Verification items for this drawing (mm, ordinates from the low corner). A direction names the side the tool comes from. Round coordinates to 2 decimals unless told otherwise and drop trailing zeros. Loops run counter-clockwise (first coordinate to the right, second up) from the corner with the lowest first, then second, coordinate; pieces in that order, holes last. Notation, with made-up numbers: (31, 5.5) - (40, 5.5) arc R33 ccw to (40, 41.5) - close; hole circle Ø6 at (39, -13). An arc over 180 degrees is marked (long way). Put each result on its own line as item: value.
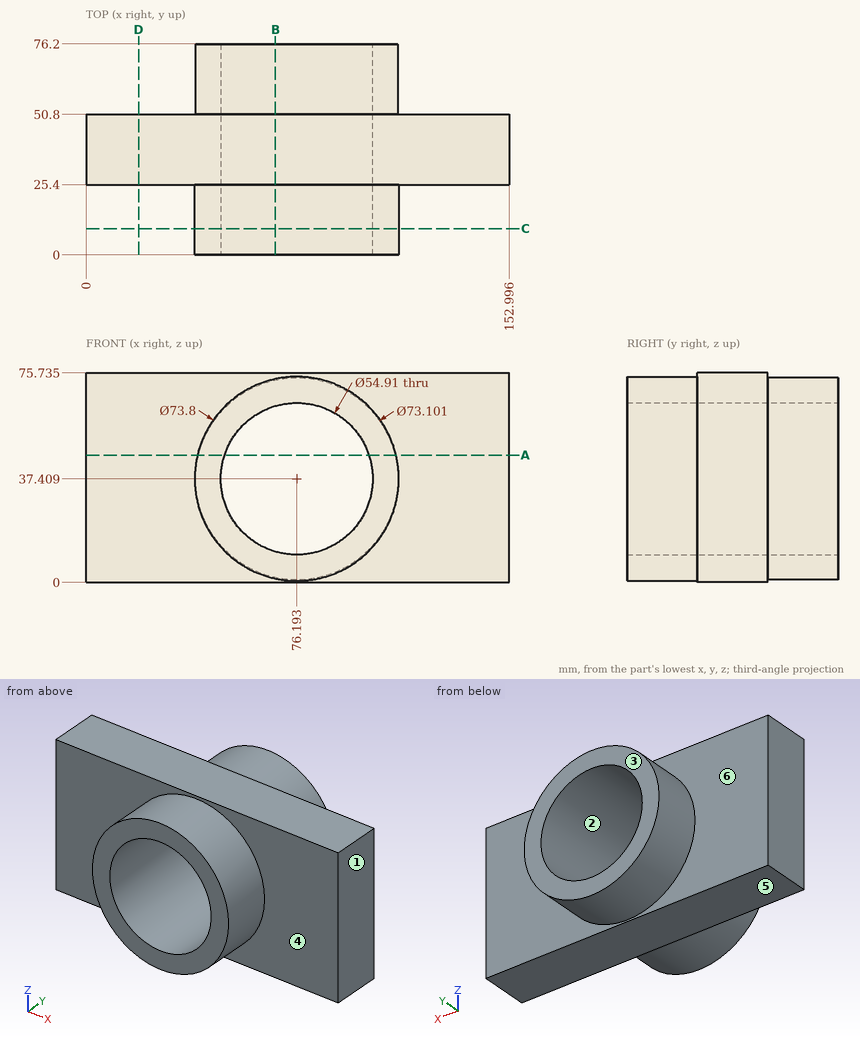
Item 1: Go/stop test with flat-tipped pins: pin 1 (12 mm diameter, centred on x = 113, z = 62, fed in from +Y); pin 2 (1.5 mm diameter, centred on y = 16, z = 49, fed in from +X) (1 decimal); pin 3 (1 mm diameter, centred on y = 38.5, z = 62.5, fed in from -X); pin 4 (12 mm diameter, centred on y = 10.5, z = 46, fed in from -X). Record where each tip stops, or that it passes through.
Filled sheet:
pin 1: y = 50.8
pin 2: x = 111.5
pin 3: x = 0
pin 4: x = 39.38
Item 2: Section check B-B on x = 68.5. Enter the section's corners in (y, z) (1 decimal).
Filled sheet:
outline: (0, 1.3) - (25.4, 1.3) - (25.4, 0) - (50.8, 0) - (50.8, 1.7) - (76.2, 1.7) - (76.2, 11.1) - (0, 11.1) - close; (0, 63.8) - (76.2, 63.8) - (76.2, 73.1) - (50.8, 73.1) - (50.8, 75.7) - (25.4, 75.7) - (25.4, 73.5) - (0, 73.5) - close
Item 3: Thickness scan on line 1 (X direction, y = 61.5, z = 52.5); line 2 (Y direction, x = 35, z = 45); line 3 (Z direction, x = 97, y = 41.5) (1 decimal). Record the ranges inside material, lowest first. Write a range as from..to.
Filled sheet:
line 1: 42.9..53.26, 99.13..109.48
line 2: 25.4..50.8
line 3: 0..19.5, 55.3..75.7
Item 4: Section check C-C on y = 9.5. Enter the section's corners in (x, z) (1 decimal), then the cut area to 3 significant figures.
Filled sheet:
outline: circle Ø73.8 at (76.2, 37.4); hole circle Ø54.9 at (76.2, 37.4)
area: 1,910 mm²
Item 5: Release check for a two-part mould opening along X. For the marked faces 1, 2 and 3 record: +X half, -X half, draft (parallel to the pull), parting line (faces both ways), or undercut.
Filled sheet:
face 1: +X half
face 2: undercut
face 3: draft
Item 6: Section check D-D on x = 19. Enter the section's corners in (y, z) (1 decimal), then the cut area to 3 significant figures.
Filled sheet:
outline: (25.4, 0) - (50.8, 0) - (50.8, 75.7) - (25.4, 75.7) - close
area: 1,920 mm²
Item 7: Tool access check on the marked faces 4, 5 and 6. Record the directions out of +Z, -Z, +X, -X, +Y, -Y that give a thin tool (end or side, any length) a straight path to the whole face; none if there is none.
Filled sheet:
face 4: -Y
face 5: -Z, +X, -X, +Y, -Y
face 6: +Y
Item 8: Section check A-A on z = 46. Enter the section's corners in (x, y).
Filled sheet:
outline: (0, 25.4) - (40.31, 25.4) - (40.31, 0) - (50.12, 0) - (50.12, 76.2) - (40.67, 76.2) - (40.67, 50.8) - (0, 50.8) - close; (102.27, 0) - (112.08, 0) - (112.08, 25.4) - (153, 25.4) - (153, 50.8) - (111.72, 50.8) - (111.72, 76.2) - (102.27, 76.2) - close
